from build123d import *

# Parameters (mm, degrees)
F1_DEPTH       = 12.5
F3_D           = 3.5
F3_CSINK_D     = 6.5
F3_CSINK_ANGLE = 70
F4_DEPTH       = 4
F5_DEPTH       = 4.5
F7_W           = 48.072574
F7_H           = 4
F8_DEPTH       = 2
F9_R           = 2
F10_DEPTH      = 19.3


with BuildPart() as f1:
    # F0 (on Top) → F1 (new body, symmetric)
    with BuildSketch(Plane.XY):
        with BuildLine():
            Line((1.472, -11.782544), (-8.527783, -11.782544))
            ThreePointArc((-8.527783, -11.782544), (-9.23489, -12.075437), (-9.527783, -12.782544))
            Line((-9.527783, -12.782544), (-9.527783, -14.782544))
            Line((-9.527783, -14.782544), (-2.527783, -14.782544))
            ThreePointArc((-2.527783, -14.782544), (-2.23489, -14.075437), (-1.527783, -13.782544))
            Line((-1.527783, -13.782544), (-1.027783, -13.782544))
            ThreePointArc((-1.027783, -13.782544), (1.447091, -14.80767), (2.472217, -17.282544))
            Line((2.472217, -17.282544), (2.472217, -31.782544))
            Line((2.472217, -31.782544), (4.472217, -31.782544))
            ThreePointArc((4.472217, -31.782544), (5.179324, -31.489651), (5.472217, -30.782544))
            Line((5.472217, -30.782544), (5.472217, -12.782544))
            ThreePointArc((5.472217, -12.782544), (5.179324, -12.075437), (4.472217, -11.782544))
            Line((4.472217, -11.782544), (1.472, -11.782544))
        make_face()
    extrude(amount=F1_DEPTH, both=True)

    # F3 (through all)
    with Locations(Plane.YZ.offset(5.472217)):
        with Locations((-25.782544, 7.5), (-25.782544, -7.5)):
            CounterSinkHole(F3_D / 2, F3_CSINK_D / 2, counter_sink_angle=F3_CSINK_ANGLE)

    # F0 (on Top) → F4 (join, symmetric)
    with BuildSketch(Plane.XY):
        with BuildLine():
            Line((-6.528, -0.913868), (-8.527783, -11.782544))
            Line((-8.527783, -11.782544), (1.472, -11.782544))
            Line((1.472, -11.782544), (1.472, 35.217456))
            ThreePointArc((1.472, 35.217456), (-0.291932, 33.74532), (-2.528, 33.217456))
            Line((-2.528, 33.217456), (-2.528, 23.217456))
            Line((-2.528, 23.217456), (-6.528, 23.217456))
            Line((-6.528, 23.217456), (-6.528, -0.913868))
        make_face()
    extrude(amount=F4_DEPTH, both=True)

    # F0 (on Top) → F5 (join, symmetric)
    with BuildSketch(Plane.XY):
        with BuildLine():
            ThreePointArc((-2.528, 33.217456), (-0.291932, 33.74532), (1.472, 35.217456))
            ThreePointArc((1.472, 35.217456), (1.944136, 40.453524), (-2.528, 43.217456))
            Line((-2.528, 43.217456), (-2.528, 41.217456))
            ThreePointArc((-2.528, 41.217456), (0.472, 38.217456), (-2.528, 35.217456))
            Line((-2.528, 35.217456), (-2.528, 33.217456))
        make_face()
    extrude(amount=F5_DEPTH, both=True)

    # F7 (on offset) → F8 (cut, symmetric)
    with BuildSketch(Plane.YZ.offset(-2.528)):
        with Locations((12.492837, 0)):
            Rectangle(F7_W, F7_H)
    extrude(amount=F8_DEPTH, both=True, mode=Mode.SUBTRACT)

    # F9 (on Front) → F10 (cut)
    with BuildSketch(Plane.XZ):
        with Locations((-2.458, 0)):
            Circle(F9_R)
    extrude(amount=F10_DEPTH, mode=Mode.SUBTRACT)


solid = f1.part
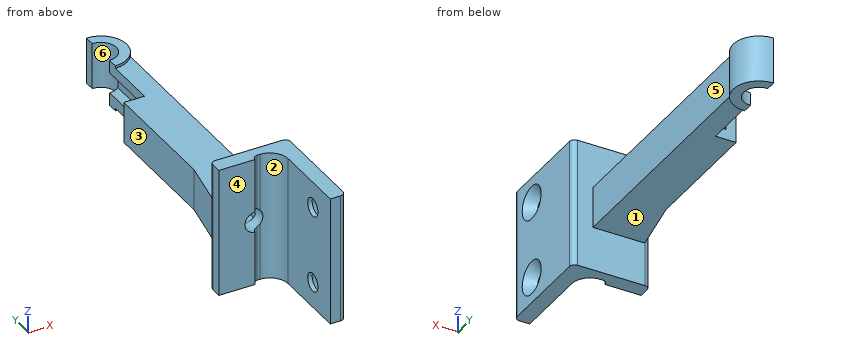
Input: part model. Units: mm. Frame: model coordinates. Face numbers are marked on the shaded views. A direction names the side the tool comes from. Give positions to 0.01 mm unless a question says otherwise; leave off trailing zeros. Loops run counter-clockwise (first coordinate to the right, second up) from the corner with the lowest first, then second, coordinate; pieces in that order, holes last. Notation, with made-up numbers: (-26.5, 2) - (5.5, 2) arc R15 ccw to (5.5, 10) - close; hole circle Ø4 at (4, 86.5). An arc over 180 degrees is marked (long way). Use CSV: the item, a comma, the result in double quotes. Start each with the question number.
Item 1: Section D-D on y = 31.5. Return loops of the section in (x, z), then the cut area to 3 significant figures.
Item 2: Section B-B on y = 9. Return loops of the section in (x, z).
Item 3: Line query: line 1 (Z direction, x = -2.75, y = 5); line 2 (Y direction, x = 2.8, z = 7.5); line 3 (X direction, y = -19.5, z = 4). Output: solid intervals per line, ascending.
Item 4: Mould query, pull axis Y, two halves, no side actions, for the marked faces 1, 2 and 3. Classes: pulls with the +Y half, pulls with the -Y half, needs draft (parallel to the pull), parting line crosses it, or undercut.
Item 5: Contact query for flat-ended pins moving along their axis: P1, Ø2.5, axis at x = 1, y = 36.5, coming from the -Z side; P2, Ø1.2, axis at y = 30.5, z = -3, coming from the -X side; P3, Ø1.2, axis at x = -1.5, z = -1.5, coming from the +Y side. Output: stop coordinate, or through.
Item 6: Section A-A on z = 7.5. Return loops of the section in (x, y), then the cut area to 3 significant figures.
Item 7: Section C-C on x = -5.5. Return loops of the section in (y, z).
Item 8: Reachability of the marked faces 4, 5 and 6 from +Z, -Z, +X, -X, +Y, -Y: full face, straight path, thin tool, end or side. Return the list, or none.
Ans:
1,outline,"(-2.53, -4) - (1.47, -4) - (1.47, 4) - (-2.53, 4) - (-2.53, 2) - (-0.53, 2) - (-0.53, -2) - (-2.53, -2) - close"
1,area,"24.0 mm2"
2,outline,"(-6.53, -4) - (1.47, -4) - (1.47, 4) - (-6.53, 4) - close; hole (-4.53, -2) - (-0.53, -2) - (-0.53, 2) - (-4.53, 2) - close"
3,line 1,"z = -4 to -2, 2 to 4"
3,line 2,"y = -31.78 to -27.53, -24.03 to -11.78"
3,line 3,"x = 2.47 to 5.47"
4,face 1,"undercut"
4,face 2,"pulls with the -Y half"
4,face 3,"needs draft"
5,P1,"stops at z = -4.5"
5,P2,"stops at x = -2.53"
5,P3,"stops at y = 43.2"
6,outline,"(-9.53, -14.78) - (-2.53, -14.78) arc R1 cw to (-1.53, -13.78) - (-1.03, -13.78) arc R3.5 cw to (2.47, -17.28) - (2.47, -24.03) - (3.33, -24.03) - (5.47, -22.53) - (5.47, -12.78) arc R1 ccw to (4.47, -11.78) - (-8.53, -11.78) arc R1 ccw to (-9.53, -12.78) - close; (2.47, -31.78) - (4.47, -31.78) arc R1 ccw to (5.47, -30.78) - (5.47, -29.03) - (3.33, -27.53) - (2.47, -27.53) - close"
6,area,"79.5 mm2"
7,outline,"(-14.78, -12.5) - (-11.78, -12.5) - (-11.78, -4) - (23.22, -4) - (23.22, 4) - (-11.78, 4) - (-11.78, 12.5) - (-14.78, 12.5) - close"
8,face 4,"+Z, -Z, -X, -Y"
8,face 5,"+Z, -Z, +X"
8,face 6,"+Z, -Z, -X"
